The model under review builds one solid part; all positions refer to its coordinate system, in mm. Coordinates: 2 decimals unless noted, no trailing zeros. Write each loop counter-clockwise with the first axis right and the second up, starting at its lowest first coordinate (ties: lowest second). Pieces come first, ordered by that corner, then holes. Notation, with made-up numbers: (-37, 55) - (-26, 55) arc R8 cw to (-26, 61) - close; hole circle Ø9 at (-19, 85.5). An arc over 180 degrees is marked (long way). Return JSON: item names as keys, results as strings. Group by question number.
(1) For pin 1 Ø2.5 at (x, z) = (15.25, 30.5) entering from +Y, flat-tipped, find the tip position at first contact; note if it passes through.
(2) We need section A-A on x = 15.25. State the section outline as (y, z) points, then the cut area to 3 significant figures.
(3) We need section B-B on z = 30.5. State the section outline as (x, y) points.
(4) To check wall thickness, follow L1, parallel to X at y = 1.05, z = 30.5; L2, parallel to Z at x = 15.5, y = 0.6; L3, parallel to Z at x = 48.5, y = 2.05. State the ranges of each line that lie inside material, in increasing order. Write a range as from..to.
```python
from build123d import *

# Parameters (mm, degrees)
SKETCH2_W               = 127
SKETCH2_H               = 127
BOSS_EXTRUDE1_DEPTH     = 3
CUT_EXTRUDE1_DEPTH      = 90.852657167
CUT_EXTRUDE1_DEPTH_BACK = 90.852657167
SKETCH3_R               = 1.5
SKETCH4_R               = 1.5
CUT_EXTRUDE2_DEPTH      = 10


with BuildPart() as part:
    # Sketch2 → Boss-Extrude1 (new body)
    with BuildSketch(Plane(origin=(0, 0, 0), x_dir=(1, 0, 0), z_dir=(0, 1, 0))):
        Rectangle(SKETCH2_W, SKETCH2_H)
    extrude(amount=BOSS_EXTRUDE1_DEPTH)

    # Sketch3 → Cut-Extrude1 (cut, two sides: drawn at the far end of the back side and taken through both)
    with BuildSketch(Plane(origin=(0, 3, 0), x_dir=(1, 0, 0), z_dir=(0, 1, 0)).offset(-CUT_EXTRUDE1_DEPTH_BACK)):
        with Locations(Location((-47.214690182, 47.214690182, 0), (0, 0, 270))):
            Circle(SKETCH3_R)
        with Locations(Location((-34.337144063, 34.337144063, 0), (0, 0, 270))):
            Circle(SKETCH3_R)
        with Locations(Location((47.214690182, 47.214690182, 0), (0, 0, 270))):
            Circle(SKETCH3_R)
        with Locations(Location((34.337144063, 34.337144063, 0), (0, 0, 270))):
            Circle(SKETCH3_R)
        with Locations(Location((47.214690182, -47.214690182, 0), (0, 0, 270))):
            Circle(SKETCH3_R)
        with Locations(Location((34.337144063, -34.337144063, 0), (0, 0, 270))):
            Circle(SKETCH3_R)
        with Locations(Location((-47.214690182, -47.214690182, 0), (0, 0, 270))):
            Circle(SKETCH3_R)
        with Locations(Location((-34.337144063, -34.337144063, 0), (0, 0, 270))):
            Circle(SKETCH3_R)
    extrude(amount=CUT_EXTRUDE1_DEPTH + CUT_EXTRUDE1_DEPTH_BACK, mode=Mode.SUBTRACT)

    # Sketch4 → Cut-Extrude2 (cut)
    with BuildSketch(Plane(origin=(0, 3, 0), x_dir=(1, 0, 0), z_dir=(0, 1, 0))):
        with Locations(Location((-15.25, 0, 0), (0, 0, 270))):
            Circle(SKETCH4_R)
        with Locations(Location((15.25, 0, 0), (0, 0, 270))):
            Circle(SKETCH4_R)
        with Locations(Location((-15.25, -30.5, 0), (0, 0, 270))):
            Circle(SKETCH4_R)
        with Locations(Location((15.25, -30.5, 0), (0, 0, 270))):
            Circle(SKETCH4_R)
    extrude(amount=-CUT_EXTRUDE2_DEPTH, mode=Mode.SUBTRACT)


solid = part.part
```
Ans:
{
 "1": {"pin 1": "through"},
 "2": {"outline": "(0, -63.5) - (3, -63.5) - (3, -1.5) - (0, -1.5) - close; (0, 1.5) - (3, 1.5) - (3, 29) - (0, 29) - close; (0, 32) - (3, 32) - (3, 63.5) - (0, 63.5) - close", "area": "363 mm²"},
 "3": {"outline": "(-63.5, 0) - (-16.75, 0) - (-16.75, 3) - (-63.5, 3) - close; (-13.75, 0) - (13.75, 0) - (13.75, 3) - (-13.75, 3) - close; (16.75, 0) - (63.5, 0) - (63.5, 3) - (16.75, 3) - close"},
 "4": {"L1": "-63.5..-16.75, -13.75..13.75, 16.75..63.5", "L2": "-63.5..-1.48, 1.48..29.02, 31.98..63.5", "L3": "-63.5..-47.99, -46.44..46.44, 47.99..63.5"}
}
